Autodesk Inventor part; units mm, degrees
ref_plane "YZ Plane" through (0, 0, 0) normal (1, 0, 0) x (0, 1, 0)
ref_plane "XZ Plane" through (0, 0, 0) normal (0, 1, 0) x (-1, 0, 0)
ref_plane "XY Plane" through (0, 0, 0) normal (0, 0, 1) x (1, 0, 0)
sketch "Sketch1" plane through (0, 0, 0) normal (0, 0, 1) x (1, 0, 0)
  line L0 (-5.4993, 0) -> (-2.7496, 4.7625)
  line L1 (-2.7496, 4.7625) -> (2.7496, 4.7625)
  line L2 (2.7496, 4.7625) -> (5.4993, 0)
  line L3 (5.4993, 0) -> (2.7496, -4.7625)
  line L4 (2.7496, -4.7625) -> (-2.7496, -4.7625)
  line L5 (-2.7496, -4.7625) -> (-5.4993, 0)
  point P0 (0, 0)
  point P1 (0, 0)
  dimension "d58" = 1.5875
  dimension "d59" = 0
  dimension "d0" = 9.525
extrude "3/8 Hex" add sketch "Sketch1" along normal blind 24.511
sketch "Sketch2" plane through (0, 0, 24.511) normal (0, 0, 1) x (1, 0, 0)
  circle A0 centre (0, 0) radius 4.7625
  dimension "d3" = 9.525
extrude "3/8 Round" add sketch "Sketch2" along normal blind 11.3347
sketch "Sketch3" plane through (0, 0, 35.8458) normal (0, 0, 1) x (1, 0, 0)
  circle A0 centre (0, 0) radius 4.7625
  circle A1 centre (0, 0) radius 3.175
  dimension "d6" = 6.35
extrude "1/4 Round" add sketch "Sketch3" along normal blind 8.6741 contours A1
sketch "Sketch7" plane through (0, 0, 0) normal (0, 0, -1) x (-1, 0, 0)
  circle A0 centre (0, 0) radius 6.35
  dimension "d18" = 12.7
extrude "1/2 Round" add sketch "Sketch7" along normal blind 7.9375
sketch "Sketch8" plane through (0, 0, -7.9375) normal (0, 0, -1) x (-1, 0, 0)
  circle A0 centre (0, 0) radius 6.35
  line L0 (-7.3323, 0) -> (-3.6662, 6.35)
  line L1 (-3.6662, 6.35) -> (3.6662, 6.35)
  line L2 (3.6662, 6.35) -> (7.3323, 0)
  line L3 (7.3323, 0) -> (3.6662, -6.35)
  line L4 (3.6662, -6.35) -> (-3.6662, -6.35)
  line L5 (-3.6662, -6.35) -> (-7.3323, 0)
  dimension "d21" = 12.7
extrude "1/2 Hex" add sketch "Sketch8" along normal blind 25.4
sketch "Sketch12" plane through (0, 0, -33.3375) normal (0, 0, -1) x (-1, 0, 0)
  circle A0 centre (0, 0) radius 5.9436
  dimension "d41" = 11.8872
extrude "Spring Clip Groove" add sketch "Sketch12" along normal blind 0.9906
sketch "Sketch13" plane through (0, 0, -34.3281) normal (0, 0, -1) x (-1, 0, 0)
  circle A0 centre (0, 0) radius 5.9436
  circle A1 centre (0, 0) radius 6.35
  dimension "d45" = 12.7
extrude "Spring Clip" add sketch "Sketch13" along normal blind 1.5875 contours A0 | A1
chamfer "Chamfer2" distance 0.7937 angle 45 1 edges at (6.35, 0, -35.9156)
sketch "Sketch14" plane through (0, 0, 35.8458) normal (0, 0, 1) x (1, 0, 0)
  circle A0 centre (0, 0) radius 3.175
  circle A1 centre (0, 0) radius 4.7625
  circle A2 centre (0, 0) radius 4.4704
  dimension "d52" = 8.9408
extrude "3/8 Spring Clip Groove" add sketch "Sketch14" along normal blind 0.7366 contours A2
sketch "Sketch15" plane through (0, 0, 36.5823) normal (0, 0, 1) x (1, 0, 0)
  circle A0 centre (0, 0) radius 3.175
  circle A1 centre (0, 0) radius 4.4704
  circle A2 centre (0, 0) radius 4.7625
  dimension "d56" = 9.525
extrude "3/8 Round 2" add sketch "Sketch15" along normal blind 1.5875 contours A1 | A2
chamfer "Chamfer3" distance 0.7937 angle 45 1 edges at (-4.7625, 0, 38.1698)
properties part number "Primary Shaft"
Read the model definition and answer for the solid it produces. Units are mm, in the model's axes. A direction names the side the tool comes from. Round coordinates to 2 decimals unless told otherwise and drop trailing zeros. Write each loop counter-clockwise with the first axis right and the second up, starting at its lowest first coordinate (ties: lowest second). Pieces come first, ordered by that corner, then holes. Notation, with made-up numbers: (-37.5, 46) - (-32.5, 46) arc R20 cw to (-32.5, 50) - close; hole circle Ø8 at (57.5, 72). An arc over 180 degrees is marked (long way). Use a Markdown table: item, result.
(1) Straight lines are drawn through the part: line 1 along Z through (x, y) = (-0.5, 5.5); line 2 along Y through (x, z) = (-0.5, 5.5); line 3 along Y through (x, z) = (6, -15.5). For each, find the intervals that lie inside material, in ascending order. Write a range as [from, to].
Reported:
| item | result |
|---|---|
| line 1 | [-35.92, 0] |
| line 2 | [-4.76, 4.76] |
| line 3 | [-2.31, 2.31] |
(2) The part is cut by section B-B (z = -28). Write down the section's boundary in (x, y), then the cut area to 3 significant figures.
Reported:
| item | result |
|---|---|
| outline | (-7.33, 0) - (-3.67, -6.35) - (3.67, -6.35) - (7.33, 0) - (3.67, 6.35) - (-3.67, 6.35) - close |
| area | 140 mm2 |
(3) The part is cut by section A-A (z = 9). Write down the section's boundary in (x, y).
Reported:
| item | result |
|---|---|
| outline | (-5.5, 0) - (-2.75, -4.76) - (2.75, -4.76) - (5.5, 0) - (2.75, 4.76) - (-2.75, 4.76) - close |
(4) Which of the six approach directions +Z, -Z, +X, -X, +Y, -Y give full straight-line access (tool end or side, diameter ignored) to faces 1 (the cylindrical face through (1.38, 6.2, -34.72)), 2 (the flat face through (-7, 0, -7.938)), 3 (the flat face through (3, -4, 24.511)), 4 (the cylindrical face through (-5.669, -1.785, -33.826))?
Reported:
| item | result |
|---|---|
| face 1 | -Z |
| face 2 | +Z, -X |
| face 3 | +Z, +X, -Y |
| face 4 | none |
(5) Each of these flat-tipped pins is pushed along its axis until it touches: pin 1 Ø4 at (x, z) = (-2, 3.5) entering from +Y; pin 2 Ø2.5 at (x, y) = (2.5, -4) entering from +Z; pin 3 Ø1 at (x, y) = (2.5, 5) entering from +Z; pin 4 Ø6 at (x, y) = (-1, -4) entering from +Z. Where does it stop, or does it pass through?
Reported:
| item | result |
|---|---|
| pin 1 | y = 4.76 |
| pin 2 | z = 38.17 |
| pin 3 | z = 24.51 |
| pin 4 | z = 44.52 |
